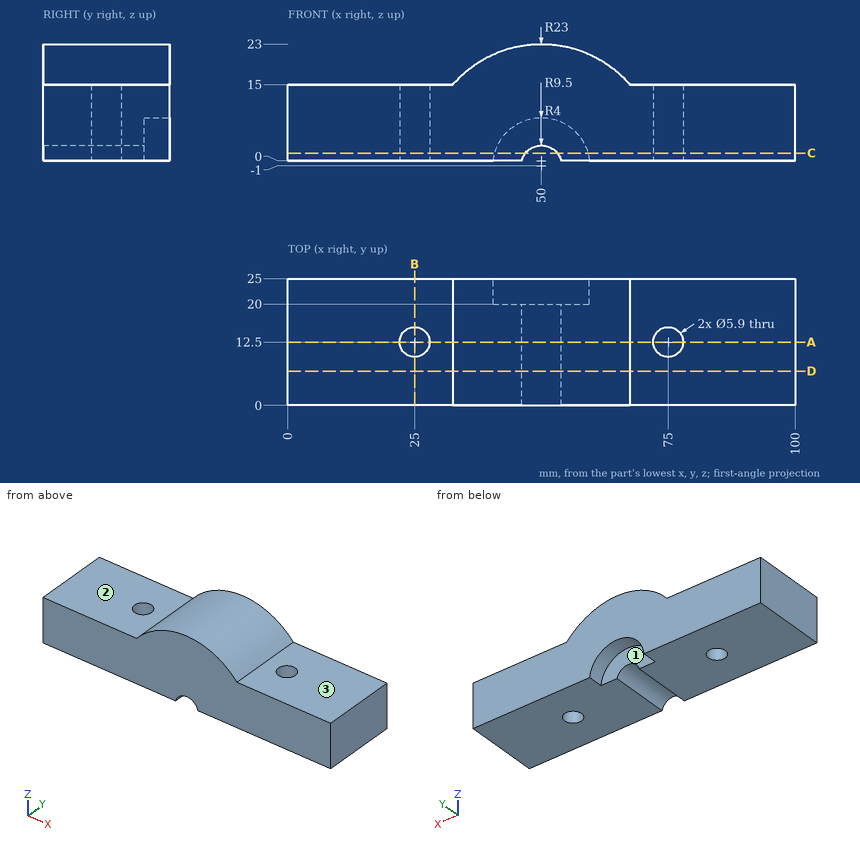
Print and shaded views of the part. All mm, measured from the part's lowest x, y and z. A direction names the side the tool comes from. Coordinates: 2 decimals unless noted, no trailing zeros. Loops run counter-clockwise (first coordinate to the right, second up) from the corner with the lowest first, then second, coordinate; pieces in that order, holes last. Notation, with made-up numbers: M -12,-24.5 L 14,-24.5 A26 ccw 14,-6.5 Z; hole C -3,71 d11. An arc over 180 degrees is marked long. Use a Markdown table: item, result. Add a question column.
Q1. Cut at B-B (x = 25). Write the cut outline in (y, z), and give its area (4 significant figures).
Q2. Probe L1, parallel to X at y = 12.5, z = 4; L2, parallel to Y at x = 75, z = 4.5; L3, parallel to X at y = 14.75, z = 6.75. List the from-to ranges inside material, lowest first.
Q3. Pin check, flat tips, straight feed: P1, Ø2, axis at x = 73.5, y = 6.5, coming from the +Z side; P2, Ø10, axis at x = 35.5, z = 19, coming from the +Y side; P3, Ø4.5, axis at x = 75, y = 12.5, coming from the +Z side; P4, Ø3, axis at y = 22, z = 17, coming from the -X side. Stop position of each tip, or through.
Q4. Cut at C-C (z = 1.5). Write the cut outline in (x, y).
Q5. Which spindle directions (+Z, -Z, +X, -X, +Y, -Y) get a long thin tool onto all of the face, cutting with end or side? Do the marked faces 1, 2 and 3. Say none if no direction does.
Q6. Cut at A-A (y = 12.5). Write the cut outline in (x, z), and give its area (3 significant figures).
Q7. Cut at D-D (y = 6.75). Write the cut outline in (x, z).
Worked out:
| question | item | result |
|---|---|---|
| 1 | outline | M 0,0 L 9.55,0 L 9.55,15 L 0,15 Z; M 15.45,0 L 25,0 L 25,15 L 15.45,15 Z |
| 1 | area | 286.5 mm2 |
| 2 | L1 | x = 0 to 22.05, 27.95 to 72.05, 77.95 to 100 |
| 2 | L2 | y = 0 to 9.55, 15.45 to 25 |
| 2 | L3 | x = 0 to 23.09, 26.91 to 73.09, 76.91 to 100 |
| 3 | P1 | stops at z = 15 |
| 3 | P2 | stops at y = 25 |
| 3 | P3 | passes through |
| 3 | P4 | stops at x = 33.01 |
| 4 | outline | M 0,0 L 46.88,0 L 46.88,20 L 40.83,20 L 40.83,25 L 0,25 Z; M 53.12,0 L 100,0 L 100,25 L 59.17,25 L 59.17,20 L 53.12,20 Z; hole C 25,12.5 d5.9; hole C 75,12.5 d5.9 |
| 5 | face 1 | -Z, +Y |
| 5 | face 2 | +Z, -X, +Y, -Y |
| 5 | face 3 | +Z, +X, +Y, -Y |
| 6 | outline | M 0,0 L 22.05,0 L 22.05,15 L 0,15 Z; M 27.95,0 L 46.13,0 A4 cw 53.87,0 L 72.05,0 L 72.05,15 L 67.44,15 A23 ccw 32.56,15 L 27.95,15 Z; M 77.95,0 L 100,0 L 100,15 L 77.95,15 Z |
| 6 | area | 1,500 mm2 |
| 7 | outline | M 0,0 L 46.13,0 A4 cw 53.87,0 L 100,0 L 100,15 L 67.44,15 A23 ccw 32.56,15 L 0,15 Z |
